from build123d import *

# Parameters (mm, degrees)
SKETCH_1_R          = 1.6
EXTRUDE_1_DEPTH     = 5.6
SKETCH_2_R          = 1.6
CUT_EXTRUDE_1_DEPTH = 65.275656356
FILLET_1_R          = 2


with BuildPart() as part:
    # ｽｹｯﾁ1 → ﾎﾞｽ - 押し出し1 (new body)
    with BuildSketch(Plane(origin=(0, 0, 0), x_dir=(1, 0, 0), z_dir=(0, 1, 0))):
        Polygon((-25, 50), (-40, 50), (-40, -50), (-25, -50), (-25, -25), (25, -25), (25, -50), (40, -50), (40, 50), (25, 50), (25, 25), (-25, 25), align=None)
        with Locations(Location((-32.5, -45, 0), (0, 0, 270))):
            Circle(SKETCH_1_R, mode=Mode.SUBTRACT)
        with Locations(Location((32.5, -45, 0), (0, 0, 270))):
            Circle(SKETCH_1_R, mode=Mode.SUBTRACT)
        with Locations(Location((-32.5, 45, 0), (0, 0, 270))):
            Circle(SKETCH_1_R, mode=Mode.SUBTRACT)
        with Locations(Location((32.5, 45, 0), (0, 0, 270))):
            Circle(SKETCH_1_R, mode=Mode.SUBTRACT)
    extrude(amount=EXTRUDE_1_DEPTH)

    # ｽｹｯﾁ2 → ｶｯﾄ - 押し出し1 (cut, through all)
    with BuildSketch(Plane(origin=(0, 5.6, 0), x_dir=(1, 0, 0), z_dir=(0, 1, 0))):
        with Locations(Location((18, 20.5, 0), (0, 0, 270))):
            Circle(SKETCH_2_R)
        with Locations(Location((18, -20.5, 0), (0, 0, 90))):
            Circle(SKETCH_2_R)
        with Locations(Location((-18, -20.5, 0), (0, 0, 270))):
            Circle(SKETCH_2_R)
        with Locations(Location((-18, 20.5, 0), (0, 0, 90))):
            Circle(SKETCH_2_R)
    extrude(amount=-CUT_EXTRUDE_1_DEPTH, mode=Mode.SUBTRACT)

    # ﾌｨﾚｯﾄ1
    fillet_1_edges = [part.edges().sort_by_distance(p)[0] for p in [
        (-25, 2.8, 50),
        (-40, 2.8, 50),
        (-40, 2.8, -50),
        (-25, 2.8, -50),
        (-25, 2.8, -25),
        (25, 2.8, -25),
        (25, 2.8, -50),
        (40, 2.8, -50),
        (40, 2.8, 50),
        (25, 2.8, 50),
        (25, 2.8, 25),
        (-25, 2.8, 25),
    ]]
    fillet(fillet_1_edges, radius=FILLET_1_R)


solid = part.part
Read the model definition and answer for the solid it produces. Units are mm, in the model's axes. A direction names the side the tool comes from. Give positions to 0.01 mm unless a question says otherwise; leave off trailing zeros. Write each loop counter-clockwise with the first axis right and the second up, starting at its lowest first coordinate (ties: lowest second). Pieces come first, ordered by that corner, then holes. Notation, with made-up numbers: (-35.75, 84) - (-10.75, 84) arc R28 cw to (-10.75, 105) - close; hole circle Ø4 at (7.5, 86). An arc over 180 degrees is marked (long way). Use CSV: the item, a comma, the result in double quotes. Start each with the question number.
(1) Consider line 1 along X through (y, z) = (3.85, 45); line 2 along X through (y, z) = (1.35, -20.5); line 3 along X through (y, z) = (5, -28). Determine where each line is inside the solid, lowest interval first.
(2) For faces 1 (the cylindrical face through (-19.586, 2.839, -20.292)), 2 (the flat face through (-25, 3, 38)), 3 (the flat face through (0, 3, -25)), determine the directions among +Z, -Z, +X, -X, +Y, -Y from which every point of the face is accessible in a straight line to the end or side of a thin tool.
(3) Find section D-D (y = 2.2). Count the separate pieces of the cut face and the enclosed holes in it, plus the area to 3 significant figures.
(4) Find section A-A (x = 32.5). Give the vertices of the cut face in (y, z), plus the area to 3 significant figures.
(5) Given P1, Ø1.7, axis at x = 10.5, y = 3.5, coming from the -Z side; P2, Ø5, axis at x = 18, z = 20.5, coming from the -Y side; P3, Ø3, axis at x = 9, y = 3, coming from the +Z side, each flat-ended and moving along its own axis, determine where each tip first touches the part or whether it passes through.
(6) Find section C-C (z = 36). Give the vertices of the cut face in (x, y).
(7) Find section B-B (z = -20.5). Give the vertices of the cut face in (x, y), plus the area to 3 significant figures.
(8) Determine the mould class of faces 4 (the cylindrical face through (-33.92, 2.76, -44.26)), 5 (the flat face through (-25, 3, -37)), 6 (the cylindrical face through (-25.6, 2.84, 49.43)) for opening direction Z: +Z half, -Z half, draft (parallel to the pull), parting line (faces both ways), or undercut.
Findings below:
1,line 1,"-40 to -34.1, -30.9 to -25, 25 to 30.9, 34.1 to 40"
1,line 2,"-40 to -19.6, -16.4 to 16.4, 19.6 to 40"
1,line 3,"-40 to -25, 25 to 40"
2,face 1,"+Y, -Y"
2,face 2,"+Z, +Y, -Y"
2,face 3,"-Z, +Y, -Y"
3,separate pieces,"1"
3,enclosed holes,"8"
3,area,"5,430 mm2"
4,outline,"(0, -50) - (5.6, -50) - (5.6, -46.6) - (0, -46.6) - close; (0, -43.4) - (5.6, -43.4) - (5.6, 43.4) - (0, 43.4) - close; (0, 46.6) - (5.6, 46.6) - (5.6, 50) - (0, 50) - close"
4,area,"524 mm2"
5,P1,"z = -25"
5,P2,"y = 0"
5,P3,"z = 25"
6,outline,"(-40, 0) - (-25, 0) - (-25, 5.6) - (-40, 5.6) - close; (25, 0) - (40, 0) - (40, 5.6) - (25, 5.6) - close"
7,outline,"(-40, 0) - (-19.6, 0) - (-19.6, 5.6) - (-40, 5.6) - close; (-16.4, 0) - (16.4, 0) - (16.4, 5.6) - (-16.4, 5.6) - close; (19.6, 0) - (40, 0) - (40, 5.6) - (19.6, 5.6) - close"
7,area,"412 mm2"
8,face 4,"undercut"
8,face 5,"draft"
8,face 6,"+Z half"
